Check sheet for the drawn part. Datum: minimum x, y, z corner. Units: mm. A direction names the side the tool comes from. Coordinates: 2 decimals unless noted, no trailing zeros. Write each loop counter-clockwise with the first axis right and the second up, starting at its lowest first coordinate (ties: lowest second). Pieces come first, ordered by that corner, then holes. Notation, with made-up numbers: (50.25, -36) -> (69.25, -36) arc R25 ccw to (69.25, -23) -> close; hole circle Ø2 at (78.5, 3.5). An arc over 180 degrees is marked (long way). Write item = value, one per line. Start each with the question number.
(1) Section check C-C (z = 33). Record the cut outline in (x, y), plus the area to 3 significant figures.
(2) Material ranges on probe 1 along X at (y, z) = (28.5, 50.5); probe 2 along X at (y, z) = (35, 43); probe 3 along Y at (x, z) = (19.5, 11.5) (1 decimal), recorded low to high. Write a range as [from, to].
(3) Gauge pin test, flat ends, axial feed: pin 1 Ø8 at (x, y) = (6.5, 36) entering from +Z (1 decimal); pin 2 Ø2 at (x, z) = (30, 34) entering from -Y; pin 3 Ø12 at (y, z) = (39, 51.5) entering from -X (1 decimal); pin 4 Ø8 at (x, y) = (20.5, 23.67) entering from -Z. Record the tip position at first contact, or that the pin passes through.
(4) Mould release check, pull along Z, two halves, no side actions. Record for the marked faces 1, 2, 3 and 4: released by +Z, released by -Z, zero draft, split by the parting line, or undercut.
(5) Section check D-D (z = 18.5). Record the cut outline in (x, y).
(6) Section check B-B (x = 22). State how many separate pieces and enclosed holes the cut face has, plus the area to 3 significant figures.
(7) Set-up check for the marked faces 5 and 6: record each of +Z, -Z, +X, -X, +Y, -Y from which the full face is reachable in a straight line by a thin tool's end or side.
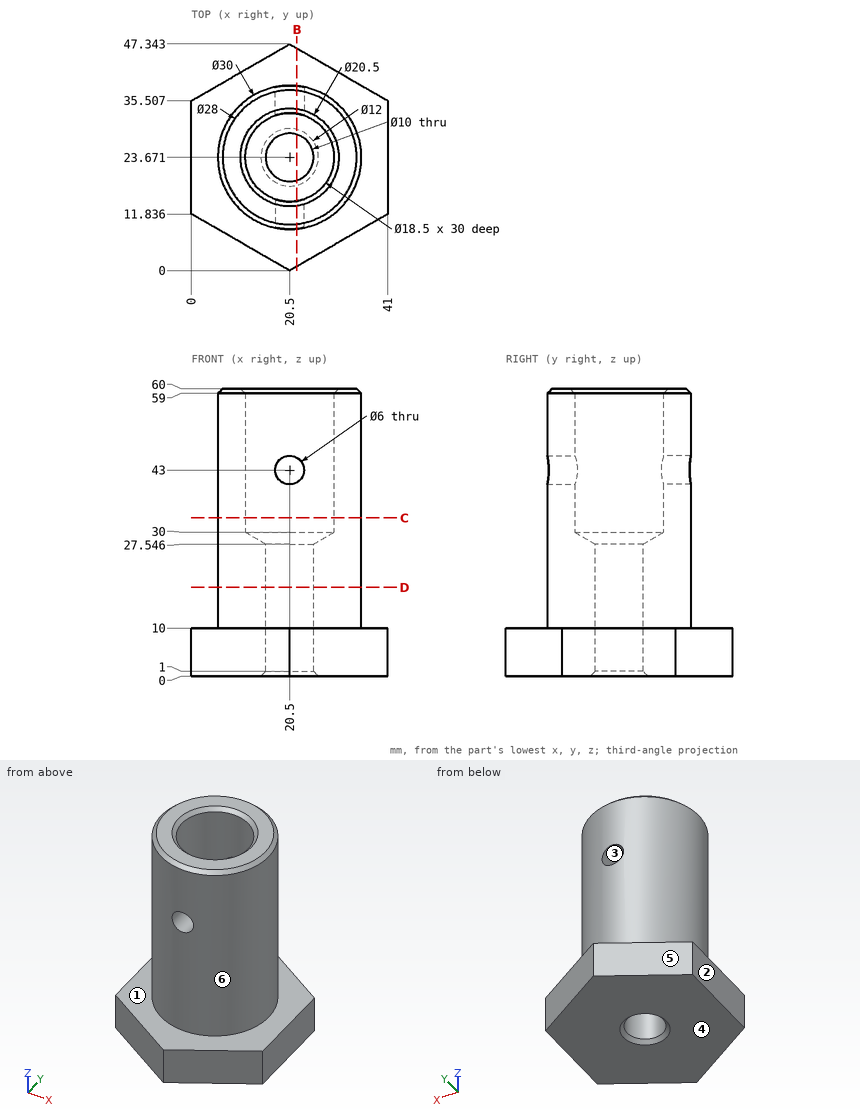
Response:
q1.outline = circle Ø30 at (20.5, 23.67); hole circle Ø18.5 at (20.5, 23.67)
q1.area = 438 mm2
q2.probe_1 = [6.3, 12.61], [28.39, 34.7]
q2.probe_2 = [10.67, 17.5], [23.5, 30.33]
q2.probe_3 = [8.7, 18.8], [28.6, 38.6]
q3.pin_1 = 59.3
q3.pin_2 = 11.31
q3.pin_3 = 8.8
q3.pin_4 = through
q4.face_1 = released by +Z
q4.face_2 = zero draft
q4.face_3 = undercut
q4.face_4 = released by -Z
q5.outline = circle Ø30 at (20.5, 23.67); hole circle Ø10 at (20.5, 23.67)
q6.separate_pieces = 4
q6.enclosed_holes = 0
q6.area = 1,040 mm2
q7.face_5 = +Z, -Z, -X, +Y
q7.face_6 = +Z
